Source: CAD feature listing. Evaluate the final solid. Frame: model axes, mm. Face numbers are marked on the shaded views. Give positions to 0.01 mm unless a question says otherwise; leave off trailing zeros. Loops run counter-clockwise (first coordinate to the right, second up) from the corner with the lowest first, then second, coordinate; pieces in that order, holes last. Notation, with made-up numbers: M 46.25,-14.5 L 79.25,-14.5 A28 ccw 79.25,9.5 Z; hole C -27,-36.5 d2. An arc over 180 degrees is marked long. Answer in a Markdown table with one row per item.
```python
from build123d import *

# Parameters (mm, degrees)
F0_W     = 38.1
F0_H     = 63.5
F1_DEPTH = 609.6


with BuildPart() as f1:
    # F0 (on Right) → F1 (new body, symmetric)
    with BuildSketch(Plane.YZ):
        with Locations((-234.823, 31.75)):
            Rectangle(F0_W, F0_H)
        Polygon((-253.873, 0), (-301.625, 0), (-301.625, -18.25625), (301.625, -18.25625), (301.625, 0), (253.873, 0), (215.773, 0), (-215.773, 0), align=None)
        with Locations((234.823, 31.75)):
            Rectangle(F0_W, F0_H)
    extrude(amount=F1_DEPTH, both=True)


solid = f1.part
```
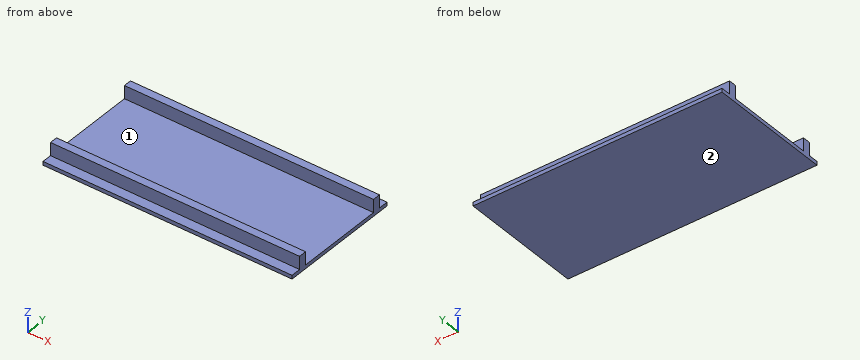
Q1. Mould query, pull axis Y, two halves, no side actions, for the marked faces 1 and 2. Classes: +Y half, -Y half, draft (parallel to the pull), parting line (faces both ways), or undercut.
Values follow:
| item | result |
|---|---|
| face 1 | undercut |
| face 2 | draft |
Q2. Ray query, probe 1 along Y at (x, z) = (-168, 35); probe 2 along Z at (x, y) = (321.5, 145.5). Return the intervals inside material, ascending. Write a range as from..to.
Values follow:
| item | result |
|---|---|
| probe 1 | -253.87..-215.77, 215.77..253.87 |
| probe 2 | -18.26..0 |
Q3. Section query A-A (z = 22.5). Output: boundary loops of the cut face in (x, y).
Values follow:
| item | result |
|---|---|
| outline | M -609.6,-253.87 L 609.6,-253.87 L 609.6,-215.77 L -609.6,-215.77 Z; M -609.6,215.77 L 609.6,215.77 L 609.6,253.87 L -609.6,253.87 Z |
Q4. Section query C-C (y = -191.5). Output: boundary loops of the cut face in (x, z), plus the area to 3 significant figures.
Values follow:
| item | result |
|---|---|
| outline | M -609.6,-18.26 L 609.6,-18.26 L 609.6,0 L -609.6,0 Z |
| area | 22,300 mm^2 |
Q5. Contact query for flat-ended pins moving along their axis: pin 1 Ø8 at (x, z) = (82.5, 39) entering from -Y; pin 2 Ø14.5 at (x, y) = (-27, -277.5) entering from +Z. Output: stop coordinate, or through.
Values follow:
| item | result |
|---|---|
| pin 1 | y = -253.87 |
| pin 2 | z = 0 |
Q6. Section query B-B (x = 216). Output: boundary loops of the cut face in (y, z) (3 decimals), plus the area to 3 significant figures.
Values follow:
| item | result |
|---|---|
| outline | M -301.625,-18.256 L 301.625,-18.256 L 301.625,0 L 253.873,0 L 253.873,63.5 L 215.773,63.5 L 215.773,0 L -215.773,0 L -215.773,63.5 L -253.873,63.5 L -253.873,0 L -301.625,0 Z |
| area | 15,900 mm^2 |
